```python
from build123d import *

# Parameters (mm, degrees)
SKETCH1_R           = 2.1
SKETCH1_W           = 25
SKETCH1_H           = 5.1
BOSS_EXTRUDE1_DEPTH = 5
CUT_EXTRUDE2_DEPTH  = 5
SKETCH4_R           = 2.1
SKETCH4_R_2         = 4
BOSS_EXTRUDE2_DEPTH = 5
SKETCH5_W           = 25.4
SKETCH5_H           = 5
SKETCH5_H_2         = 5.4
CUT_EXTRUDE3_DEPTH  = 10
BOSS_EXTRUDE3_DEPTH = 5
SKETCH7_R           = 8
CUT_EXTRUDE6_DEPTH  = 5


with BuildPart() as part:
    # Sketch1 → Boss-Extrude1 (new body)
    with BuildSketch(Plane.XY):
        with BuildLine():
            Line((-65, 61.5), (0, 61.5))
            Line((0, 61.5), (0, 0))
            Line((0, 0), (-1.877501001, 0))
            ThreePointArc((-1.877501001, 0), (-5, -1.5), (-8.122498999, 0))
            Line((-8.122498999, 0), (-20, 0))
            Line((-20, 0), (-20, 5))
            Line((-20, 5), (-45, 5))
            Line((-45, 5), (-45, 0))
            Line((-45, 0), (-56.877501001, 0))
            ThreePointArc((-56.877501001, 0), (-60, -1.5), (-63.122498999, 0))
            Line((-63.122498999, 0), (-65, 0))
            Line((-65, 0), (-65, 61.5))
        make_face()
        with Locations((-60, 56.5)):
            Circle(SKETCH1_R, mode=Mode.SUBTRACT)
        with Locations((-5, 56.5)):
            Circle(SKETCH1_R, mode=Mode.SUBTRACT)
        with Locations((-60, 46.5)):
            Circle(SKETCH1_R, mode=Mode.SUBTRACT)
        with Locations((-5, 46.5)):
            Circle(SKETCH1_R, mode=Mode.SUBTRACT)
        with Locations(Location((-5, 12.5, 0), (0, 0, 180))):
            Circle(SKETCH1_R, mode=Mode.SUBTRACT)
        with Locations(Location((-5, 2.5, 0), (0, 0, 180))):
            Circle(SKETCH1_R, mode=Mode.SUBTRACT)
        with Locations(Location((-60, 2.5, 0), (0, 0, 180))):
            Circle(SKETCH1_R, mode=Mode.SUBTRACT)
        with Locations(Location((-60, 12.5, 0), (0, 0, 180))):
            Circle(SKETCH1_R, mode=Mode.SUBTRACT)
        with Locations((-32.5, 12.5)):
            Rectangle(SKETCH1_W, SKETCH1_H, mode=Mode.SUBTRACT)
    extrude(amount=BOSS_EXTRUDE1_DEPTH)

    # Sketch3 → Cut-Extrude2 (cut)
    with BuildSketch(Plane(origin=(0, 0, 0), x_dir=(-1, 0, 0), z_dir=(0, 0, -1))):
        with BuildLine():
            Line((41, 15.05), (41, 34.55))
            ThreePointArc((41, 34.55), (26, 49.55), (11, 34.55))
            Line((11, 34.55), (11, 15.05))
            Line((11, 15.05), (41, 15.05))
        make_face()
    extrude(amount=-CUT_EXTRUDE2_DEPTH, mode=Mode.SUBTRACT)

    # Sketch4 → Boss-Extrude2 (add)
    with BuildSketch(Plane(origin=(0, 0, 0), x_dir=(-1, 0, 0), z_dir=(0, 0, -1))):
        Polygon((0, 41.5), (-17.5, 63.5), (-17.5, 77.5), (65, 77.5), (65, 61.5), (0, 61.5), align=None)
        with Locations((-11.5, 69.5)):
            Circle(SKETCH4_R, mode=Mode.SUBTRACT)
        with Locations((13.5, 69.5)):
            Circle(SKETCH4_R, mode=Mode.SUBTRACT)
        with Locations((26, 69.5)):
            Circle(SKETCH4_R_2, mode=Mode.SUBTRACT)
        with Locations((38.5, 69.5)):
            Circle(SKETCH4_R, mode=Mode.SUBTRACT)
    extrude(amount=-BOSS_EXTRUDE2_DEPTH)

    # Sketch5 → Cut-Extrude3 (cut)
    with BuildSketch(Plane(origin=(0, 0, 0), x_dir=(-1, 0, 0), z_dir=(0, 0, -1))):
        with Locations((32.5, 2.5)):
            Rectangle(SKETCH5_W, SKETCH5_H)
        with Locations((32.5, 12.55)):
            Rectangle(SKETCH5_W, SKETCH5_H_2)
    extrude(amount=-CUT_EXTRUDE3_DEPTH, mode=Mode.SUBTRACT)

    # Sketch6 → Boss-Extrude3 (add)
    with BuildSketch(Plane(origin=(0, 0, 0), x_dir=(-1, 0, 0), z_dir=(0, 0, -1))):
        with BuildLine():
            Line((17.05572809, 77.5), (34.94427191, 77.5))
            ThreePointArc((34.94427191, 77.5), (26, 81.5), (17.05572809, 77.5))
        make_face()
    extrude(amount=-BOSS_EXTRUDE3_DEPTH)

    # Sketch7 → Cut-Extrude6 (cut)
    with BuildSketch(Plane(origin=(0, 0, 0), x_dir=(-1, 0, 0), z_dir=(0, 0, -1))):
        with Locations((26, 69.5)):
            Circle(SKETCH7_R)
    extrude(amount=-CUT_EXTRUDE6_DEPTH, mode=Mode.SUBTRACT)


solid = part.part
```
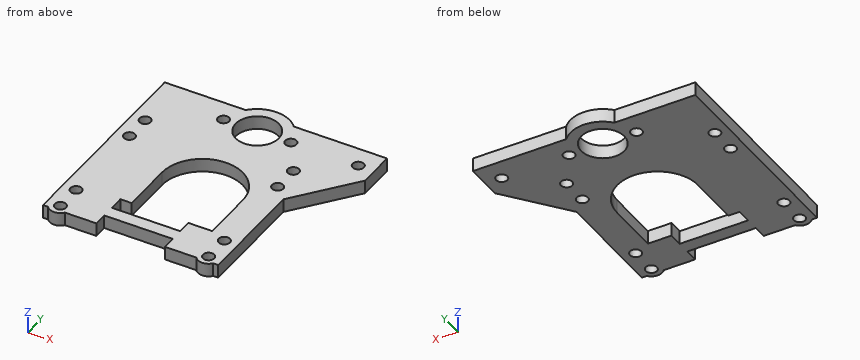
Can you work these out from the model? Positions are in its coordinate system, mm. Coordinates: 2 decimals unless noted, no trailing zeros. Write each loop counter-clockwise with the first axis right and the second up, starting at its lowest first coordinate (ties: lowest second). Pieces come first, ordered by that corner, then holes. Notation, with made-up numbers: (2, 89.5) - (31, 89.5) arc R26 cw to (31, 110.5) - close; hole circle Ø8 at (-25, 2). An arc over 180 degrees is marked (long way). Return JSON: item names as keys, results as strings.
Q1. If we section it at A-A (y = 69.5): Please give me the cut outline in (x, z).
Computed values:
{"outline": "(-65, 0) - (-40.6, 0) - (-40.6, 5) - (-65, 5) - close; (-36.4, 0) - (-34, 0) - (-34, 5) - (-36.4, 5) - close; (-18, 0) - (-15.6, 0) - (-15.6, 5) - (-18, 5) - close; (-11.4, 0) - (9.4, 0) - (9.4, 5) - (-11.4, 5) - close; (13.6, 0) - (17.5, 0) - (17.5, 5) - (13.6, 5) - close"}
Q2. If we section it at B-B (x = -60): Please give me the cut outline in (y, z), then the cut area to 3 significant figures.
Computed values:
{"outline": "(-1.5, 0) - (0.4, 0) - (0.4, 5) - (-1.5, 5) - close; (4.6, 0) - (10.4, 0) - (10.4, 5) - (4.6, 5) - close; (14.6, 0) - (44.4, 0) - (44.4, 5) - (14.6, 5) - close; (48.6, 0) - (54.4, 0) - (54.4, 5) - (48.6, 5) - close; (58.6, 0) - (77.5, 0) - (77.5, 5) - (58.6, 5) - close", "area": "311 mm2"}
Q3. I'm going to push flat-ended pins straight in: pin 1 Ø6.5 at (x, y) = (-13.5, 69.5) entering from -Z; pin 2 Ø2 at (x, z) = (-1, 2.5) entering from -Y; pin 3 Ø1.5 at (x, z) = (-53, 3.5) entering from -Y; pin 4 Ø1.5 at (x, z) = (-16, 1.5) entering from +Y. Where does each tip first touch, or does it pass through?
Computed values:
{"pin 1": "stops at z = 0", "pin 2": "stops at y = -0.15", "pin 3": "stops at y = 0", "pin 4": "stops at y = 77.5"}
Q4. If we section it at D-D (y = 56.5): Please give me the cut outline in (x, z), then the cut area to 3 significant figures.
Computed values:
{"outline": "(-65, 0) - (-62.1, 0) - (-62.1, 5) - (-65, 5) - close; (-57.9, 0) - (-7.1, 0) - (-7.1, 5) - (-57.9, 5) - close; (-2.9, 0) - (11.93, 0) - (11.93, 5) - (-2.9, 5) - close", "area": "343 mm2"}
Q5. Please list where these lines run through material, in increasing order: L1, parallel to Y at x = -26, z = 3.35; L2, parallel to X at y = 12.5, z = 3.85; L3, parallel to Y at x = -60, z = 2.85. Write a range as from..to.
Computed values:
{"L1": "y = 5..9.85, 49.55..61.5, 77.5..81.5", "L2": "x = -65..-62.1, -57.9..-45.2, -19.8..-7.1, -2.9..0", "L3": "y = -1.5..0.4, 4.6..10.4, 14.6..44.4, 48.6..54.4, 58.6..77.5"}
Q6. If we section it at C-C (y = 18.5): Please give me the cut outline in (x, z), then the cut area to 3 significant figures.
Computed values:
{"outline": "(-65, 0) - (-41, 0) - (-41, 5) - (-65, 5) - close; (-11, 0) - (0, 0) - (0, 5) - (-11, 5) - close", "area": "175 mm2"}
